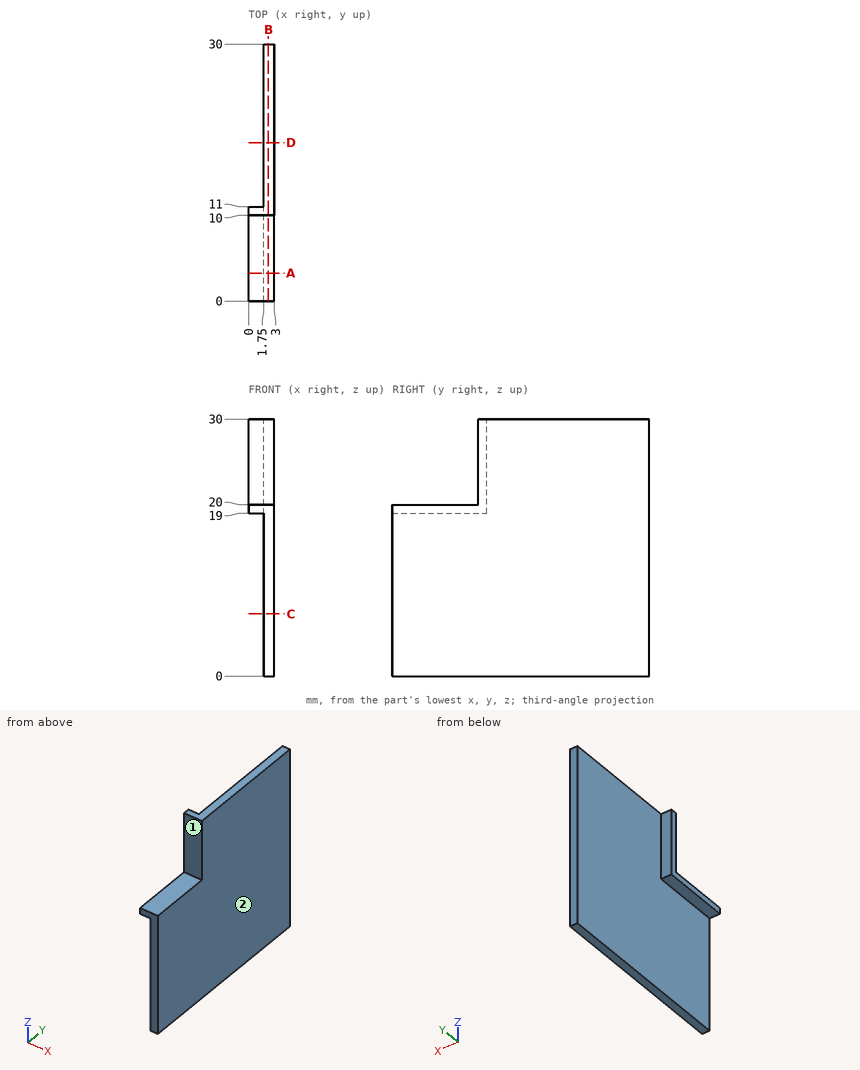
Input: dimensioned drawing with shaded views. Units: mm. Origin: part minimum x, y, z. A direction names the side the tool comes from. Coordinates: 2 decimals unless noted, no trailing zeros. Order: outer loops, then holes, each group sorted by start corner. A loop starts at its lowest first (then second) coordinate and runs counter-clockwise, first axis right, second up. Notation, with made-up numbers: (-17.5, 3) -> (33.5, 3) arc R31 ccw to (33.5, 32) -> close; hole circle Ø5 at (42.25, 44.5). An arc over 180 degrees is marked (long way). Answer in a Markdown table with one row per item.
Item 1: Contact query for flat-ended pins moving along their axis: P1, Ø1.5, axis at x = 2, y = 4.5, coming from the +Z side; P2, Ø1, axis at y = 22.5, z = 18.5, coming from the -X side; P3, Ø0.9, axis at x = 1.5, z = 23.5, coming from the -Y side. Output: stop coordinate, or through.
Return value:
| item | result |
|---|---|
| P1 | stops at z = 20 |
| P2 | stops at x = 1.75 |
| P3 | stops at y = 10 |
Item 2: Access query for the marked faces 1 and 2. Directions: +Z, -Z, +X, -X, +Y, -Y. A direction counts if a zero-diameter tool reaches every point of the face in a straight line with its end or side. Return the directions, or none.
Return value:
| item | result |
|---|---|
| face 1 | +Z, +X, -X, -Y |
| face 2 | +Z, -Z, +X, +Y, -Y |
Item 3: Ray query, L1, parallel to Y at x = 1.6, z = 28.5; L2, parallel to X at y = 26.25, z = 9.5; L3, parallel to Y at x = 1.9, z = 22.25. Return the intervals inside material, ascending.
Return value:
| item | result |
|---|---|
| L1 | y = 10 to 11 |
| L2 | x = 1.75 to 3 |
| L3 | y = 10 to 30 |
Item 4: Section A-A on y = 3.25. Output: boundary loops of the cut face in (x, z).
Return value:
| item | result |
|---|---|
| outline | (0, 19) -> (1.75, 19) -> (1.75, 0) -> (3, 0) -> (3, 20) -> (0, 20) -> close |
Item 5: Section B-B on x = 2.3. Output: boundary loops of the cut face in (y, z), plus the area to 3 significant figures.
Return value:
| item | result |
|---|---|
| outline | (0, 0) -> (30, 0) -> (30, 30) -> (10, 30) -> (10, 20) -> (0, 20) -> close |
| area | 800 mm² |
Item 6: Section C-C on z = 7.25. Output: boundary loops of the cut face in (x, y).
Return value:
| item | result |
|---|---|
| outline | (1.75, 0) -> (3, 0) -> (3, 30) -> (1.75, 30) -> close |
